```python
from build123d import *

# Parameters (mm, degrees)
ESQUISSE1_W        = 70
ESQUISSE1_H        = 22.5
ESQUISSE1_R        = 7.5
ESQUISSE1_R_2      = 1.5
BOSS_EXTRU_1_DEPTH = 5


with BuildPart() as part:
    # Esquisse1 → Boss.-Extru.1 (new body)
    with BuildSketch(Plane.XY):
        with Locations((0, 1.25)):
            Rectangle(ESQUISSE1_W, ESQUISSE1_H)
        Circle(ESQUISSE1_R, mode=Mode.SUBTRACT)
        with Locations((30, -5)):
            Circle(ESQUISSE1_R_2, mode=Mode.SUBTRACT)
        with Locations((30, 5)):
            Circle(ESQUISSE1_R_2, mode=Mode.SUBTRACT)
        with Locations((-30, 5)):
            Circle(ESQUISSE1_R_2, mode=Mode.SUBTRACT)
        with Locations((-30, -5)):
            Circle(ESQUISSE1_R_2, mode=Mode.SUBTRACT)
    extrude(amount=BOSS_EXTRU_1_DEPTH)


solid = part.part
```
Verification items for the finished model (mm, model axes). Coordinates: 2 decimals unless noted, no trailing zeros. Write each loop counter-clockwise with the first axis right and the second up, starting at its lowest first coordinate (ties: lowest second). Pieces come first, ordered by that corner, then holes. Notation, with made-up numbers: M 69,76.5 L 108,76.5 A32 ccw 108,109.5 Z; hole C 88.5,72.5 d6. An arc over 180 degrees is marked long. One line per item, written item: value.
Item 1: Section check A-A, the plane x = 30. Record the boundary of the cut face in (y, z).
Check sheet entries:
outline: M -10,0 L -6.5,0 L -6.5,5 L -10,5 Z; M -3.5,0 L 3.5,0 L 3.5,5 L -3.5,5 Z; M 6.5,0 L 12.5,0 L 12.5,5 L 6.5,5 Z
Item 2: Section check C-C, the plane z = 3.45. Record the boundary of the cut face in (x, y).
Check sheet entries:
outline: M -35,-10 L 35,-10 L 35,12.5 L -35,12.5 Z; hole C -30,-5 d3; hole C -30,5 d3; hole C 0,0 d15; hole C 30,-5 d3; hole C 30,5 d3
Item 3: Section check D-D, the plane y = -2.5. Record the boundary of the cut face in (x, z).
Check sheet entries:
outline: M -35,0 L -7.07,0 L -7.07,5 L -35,5 Z; M 7.07,0 L 35,0 L 35,5 L 7.07,5 Z
Item 4: Mould release check, pull along Y, two halves, no side actions. Record for faces 1 (the cylindrical face through (-31.5, 5.07, 2.46)), 2 (the flat face through (-35, 1, 2)), 3 (the flat face through (0, 12.5, 2)): pulls with the +Y half, pulls with the -Y half, needs draft (parallel to the pull), parting line crosses it, or undercut.
Check sheet entries:
face 1: undercut
face 2: needs draft
face 3: pulls with the +Y half
Item 5: Gauge pin test, flat end, axial feed: pin 1 Ø4 at (x, y) = (-30, 5) entering from -Z. Record the tip position at first contact, or that the pin passes through.
Check sheet entries:
pin 1: stops at z = 0
Item 6: Section check B-B, the plane x = 0. Record the boundary of the cut face in (y, z).
Check sheet entries:
outline: M -10,0 L -7.5,0 L -7.5,5 L -10,5 Z; M 7.5,0 L 12.5,0 L 12.5,5 L 7.5,5 Z
Item 7: Scan lines: line 1 along Y through (x, z) = (-30, 3.9); line 2 along Y through (x, z) = (0, 1.8); line 3 along Y through (x, z) = (29, 2.1). Record each from-to range of solid material in increasing order.
Check sheet entries:
line 1: y = -10 to -6.5, -3.5 to 3.5, 6.5 to 12.5
line 2: y = -10 to -7.5, 7.5 to 12.5
line 3: y = -10 to -6.12, -3.88 to 3.88, 6.12 to 12.5
